Autodesk Fusion 360 part; units mm, degrees
sketch "Sorted Smarties Cover Connector Base" plane through (0, 0, 0) normal (0, 0, 1) x (1, 0, 0)
  line L0 (0, 0) -> (30, 0)
  line L1 (30, 0) -> (30, 15)
  line L2 (30, 15) -> (0, 15)
  line L3 (0, 15) -> (0, 0)
  dimension "d5" = 15
  dimension "d6" = 30
extrude "Extrude1" add sketch "Sorted Smarties Cover Connector Base" along normal blind 15
sketch "Connecting Section" plane through (0, 0, 15) normal (0, 0, 1) x (-1, 0, 0)
  line L0 (0, -15) -> (0, 0)
  line L1 (0, 0) -> (-30, 0)
  line L2 (-30, 0) -> (-30, -15)
  line L3 (-30, -15) -> (0, -15)
  line L4 (-30, -11) -> (-4, -11)
  line L5 (-4, -11) -> (-4, -4)
  line L6 (-4, -4) -> (-30, -4)
  line L7 (-30, -4) -> (-30, -11)
  dimension "d7" = 7
  dimension "d8" = 4
  dimension "d9" = 4
  dimension "d10" = 4
extrude "Extrude2" cut sketch "Connecting Section" against normal blind 11 contours L2 L4 L5 L6 L7
equation "d8 = ( ( 15 - 7 ) / 2 ) * 1 mm"
Could you check a few things on this model? Use its own coordinates, in mm. A direction names the side the tool comes from. Give positions to 0.01 mm unless a question says otherwise; leave off trailing zeros. Order: outer loops, then holes, each group sorted by start corner. A loop starts at its lowest first (then second) coordinate and runs counter-clockwise, first axis right, second up.
Q1. Suppose I cut it at B-B, the plane x = 10.75. Write out the boundary of the cut face in (y, z), and give its area (3 significant figures).
Q2. I'm going to push flat-ended pins straight in: P1, Ø6, axis at y = 9.5, z = 9.5, coming from the +X side; P2, Ø2, axis at y = 6, z = 8.5, coming from the +X side. Where does each tip first touch, or does it pass through?
Q3. Suppose I cut it at C-C, the plane y = 7.5. Write out the boundary of the cut face in (x, z).
Q4. We'd pull the mould along Y, two halves only. Please class faces 3 (the flat face through (15, 0, 7)), 4 (the flat face through (17, 4, 10)), 5 (the flat face through (15, 8, 0)): +Y half, -Y half, draft (parallel to the pull), parting line (faces both ways), or undercut.
Q5. If I drill on line 1 along Y through (x, z) = (24.75, 11.5); line 2 along X through (y, z) = (10, 9.25), over which ranges is the centre line in solid material (lowest first)?
Q6. Suppose I cut it at A-A, the plane z = 6.25. Write out the boundary of the cut face in (x, y), and give its area (3 significant figures).
Q7. For faces 1 (the flat face through (17, 11, 10)), 2 (the flat face through (30, 7, 2)), which set-ups out of +Z, -Z, +X, -X, +Y, -Y let a thin tool reach every point of the face, with its end or its side?
Solution:
1. outline: (0, 0) - (15, 0) - (15, 15) - (11, 15) - (11, 4) - (4, 4) - (4, 15) - (0, 15) - close
1. area: 148 mm2
2. P1: stops at x = 30
2. P2: stops at x = 4
3. outline: (0, 0) - (30, 0) - (30, 4) - (4, 4) - (4, 15) - (0, 15) - close
4. face 3: -Y half
4. face 4: undercut
4. face 5: draft
5. line 1: y = 0 to 4, 11 to 15
5. line 2: x = 0 to 4
6. outline: (0, 0) - (30, 0) - (30, 4) - (4, 4) - (4, 11) - (30, 11) - (30, 15) - (0, 15) - close
6. area: 268 mm2
7. face 1: +Z, +X
7. face 2: +Z, -Z, +X, +Y, -Y
